Autodesk Inventor part; units mm, degrees
ref_plane "Work Plane2" through (-3.375, 53.625, 0) normal (0, 0, 1) x (1, 0, 0)
ref_plane "YZ Plane" through (0, 0, 0) normal (1, 0, 0) x (0, 1, 0)
ref_plane "XZ Plane" through (0, 0, 0) normal (0, 1, 0) x (-1, 0, 0)
ref_plane "Work Plane1" through (0, 0, 15) normal (0, 0, 1) x (1, 0, 0)
sketch "Sketch1" plane through (0, 0, 15) normal (0, 0, 1) x (1, 0, 0)
  circle A0 centre (0, 64) radius 1.4
  circle A1 centre (0, 0) radius 1.4
  circle A2 centre (38.4621, 0) radius 1.4
  circle A3 centre (76.9242, 0) radius 1.4
  circle A4 centre (76.9242, 64) radius 1.4
  circle A5 centre (38.4621, 64) radius 1.4
  circle A6 centre (-0.5, 56.5) radius 1.375
  circle A7 centre (-0.5, 7.5) radius 1.375
  circle A8 centre (57.5, 7.5) radius 1.375
  circle A9 centre (57.5, 56.5) radius 1.375
  line L0 (0, 68) -> (76.9242, 68)
  arc A10 (80.9242, 64) -> (76.9242, 68) centre (76.9242, 64) ccw
  line L1 (80.9242, 64) -> (80.9242, 0)
  arc A11 (76.9242, -4) -> (80.9242, 0) centre (76.9242, 0) ccw
  line L2 (76.9242, -4) -> (0, -4)
  arc A12 (-4, 0) -> (0, -4) centre (0, 0) ccw
  line L3 (-4, 0) -> (-4, 64)
  arc A13 (0, 68) -> (-4, 64) centre (0, 64) ccw
  line L4 (57.5, 60.619) -> (2.1636, 60.619)
  line L5 (2.1636, 60.619) -> (2.1636, 51.644)
  line L6 (2.1636, 51.644) -> (57.5, 51.644)
  line L7 (57.5, 51.644) -> (57.5, 60.619)
  line L8 (80.9242, 59.8893) -> (61.2665, 59.8893)
  line L9 (61.2665, 59.8893) -> (61.2665, 4.7989)
  line L10 (61.2665, 4.7989) -> (80.9242, 4.7989)
  line L11 (80.9242, 4.7989) -> (80.9242, 59.8893)
  point P0 (0, 0)
extrude "Extrusion1" add sketch "Sketch1" against normal blind 2 contours A6 | A7 | A8 | A9 L7 | L7 A9 | L0 A10 L1 L8 L9 L10 A11 L2 A12 L3 A13
sketch "Sketch2" plane through (0, 0, 13) normal (0, 0, -1) x (-1, 0, 0)
  circle A0 centre (-38.4621, 0) radius 2.9
  circle A1 centre (-38.4621, 64) radius 2.9
  circle A2 centre (0, 0) radius 1.4
  circle A3 centre (-38.4621, 0) radius 1.4
  circle A4 centre (-76.9242, 0) radius 1.4
  circle A5 centre (-76.9242, 64) radius 1.4
  circle A6 centre (-38.4621, 64) radius 1.4
  circle A7 centre (0, 64) radius 1.4
  circle A8 centre (-76.9242, 0) radius 4
  circle A9 centre (-76.9242, 64) radius 4
  circle A10 centre (0, 64) radius 4
  circle A11 centre (0, 0) radius 4
  point P0 (0, 0)
ref_plane "Work Plane2" through (-3.375, 53.625, 0) normal (0, 0, 1) x (1, 0, 0)
extrude "Extrusion2" add sketch "Sketch2" along normal up to surface (13 mm away)
fillet "Fillet1" radius 4 4 edges at (61.2665, 4.7989, 14) (61.2665, 59.8893, 14) (80.9242, 59.8893, 14) (80.9242, 4.7989, 14)
sketch "Sketch3" plane through (0, 0, 15) normal (0, 0, 1) x (1, 0, 0)
  circle A0 centre (46, 6.6021) radius 1.05
  line L0 (48, 30.0021) -> (-9, 30.0021)
  line L1 (-9, 30.0021) -> (-9, 4.6021)
  line L2 (-9, 4.6021) -> (48, 4.6021)
  line L3 (48, 4.6021) -> (48, 30.0021)
  circle A1 centre (-1, 27.9021) radius 1.05
  circle A2 centre (46, 6.6021) radius 1.05
  circle A3 centre (46, 28.0021) radius 1.05
  circle A4 centre (-0.5, 7.5) radius 1.375
  line L4 (43.458, 3.7531) -> (1.4128, 3.7531)
  line L5 (1.4128, 3.7531) -> (1.4128, 8.2423)
  line L6 (1.4128, 8.2423) -> (43.458, 8.2423)
  line L7 (43.458, 8.2423) -> (43.458, 3.7531)
  line L8 (43.458, 31.4547) -> (0.5917, 31.4547)
  line L9 (0.5917, 31.4547) -> (0.5917, 25.5421)
  line L10 (0.5917, 25.5421) -> (43.458, 25.5421)
  line L11 (43.458, 25.5421) -> (43.458, 31.4547)
  point P0 (0, 0)
extrude "Extrusion3" cut sketch "Sketch3" against normal through all contours A0 | L11 L10 L9 L0 | L0 L9 L8 L11 | L7 L4 L5 L2 | L2 L5 L6 L7 | A3
sketch "Sketch4" plane through (0, 0, 15) normal (0, 0, 1) x (1, 0, 0)
  line L0 (76.9242, 68) -> (0, 68)
  line L1 (-4, 64) -> (-4, 0)
  point P0 (0, 0)
  point P1 (28, 63.5)
  point P2 (54, 33.5)
  dimension "d8" = 4.5
  dimension "d9" = 32
  dimension "d10" = 30
  dimension "d11" = 26
hole "Hole1" at (28, 63.5, 15) at (54, 33.5, 15) direction (0, 0, -1) diameter 2.8 depth 20 tip angle 118
properties part number "cellSTORM_v5_Electronicbox_midlayer"
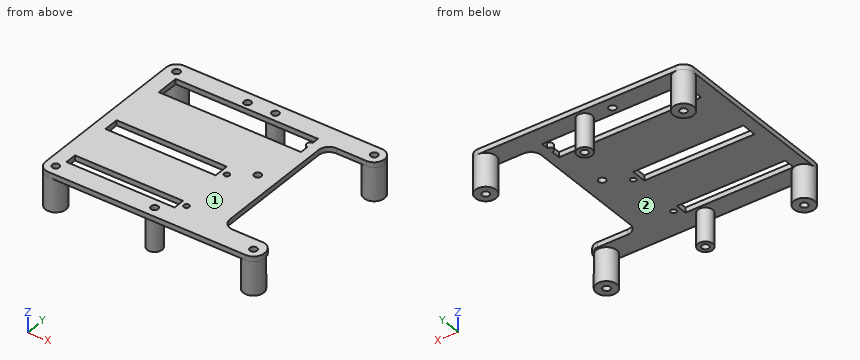
Build history of the part. All positions in model axes, mm. Face numbers are marked on the shaded views. Coordinates: 2 decimals unless noted, no trailing zeros. Write each loop counter-clockwise with the first axis right and the second up, starting at its lowest first coordinate (ties: lowest second). Pieces come first, ordered by that corner, then holes.
(1) Cut at C-C on x = 54. List the corners of the cut face in (y, z), and give its area (3 significant figures).
(2) Pin check, flat tips, straight feed: pin 1 Ø2.5 at (x, y) = (38.46, 64) entering from +Z; pin 2 Ø8 at (x, y) = (52, 20.5) entering from -Z; pin 3 Ø1.6 at (y, z) = (7, 13.5) entering from +X; pin 4 Ø1 at (y, z) = (54, 13.5) entering from +X. Stop position of each tip, or through.
(3) Drill centre lines: line 1 (Y direction, x = 0, z = 13.5); line 2 (X direction, y = 0, z = 13.65); line 3 (Y direction, x = 46, z = 14). Where is each one in solid material? Low to high.
(4) Cut at B-B on z = 7.5. State how many separate pieces and enclosed holes the cut face has, and give its area (3 significant figures).
(5) Cut at D-D on x = 12. List the corners of the cut face in (y, z), and give its area (3 significant figures).
(6) Mould opens along Y. For the marked faces 1 and 2 say: pulls with the +Y half, pulls with the -Y half, needs draft (parallel to the pull), parting line crosses it, or undercut.
(7) Cut at A-A on x = 28. List the corners of the cut face in (y, z), and give its area (3 significant figures).
Working result:
1. outline: (-4, 13) - (32.1, 13) - (32.1, 15) - (-4, 15) - close; (34.9, 13) - (51.64, 13) - (51.64, 15) - (34.9, 15) - close; (60.62, 13) - (68, 13) - (68, 15) - (60.62, 15) - close
1. area: 120 mm2
2. pin 1: passes through
2. pin 2: stops at z = 13
2. pin 3: stops at x = 62.23
2. pin 4: stops at x = 61.27
3. line 1: y = -4 to -1.4, 1.4 to 62.6, 65.4 to 68
3. line 2: x = -4 to -1.4, 1.4 to 37.06, 39.86 to 75.52, 78.32 to 80.92
3. line 3: y = -4 to 5.55, 7.65 to 26.95, 29.05 to 51.64, 60.62 to 68
4. separate pieces: 6
4. enclosed holes: 6
4. area: 217 mm2
5. outline: (-4, 13) - (3.75, 13) - (3.75, 15) - (-4, 15) - close; (8.24, 13) - (25.54, 13) - (25.54, 15) - (8.24, 15) - close; (31.45, 13) - (51.64, 13) - (51.64, 15) - (31.45, 15) - close; (60.62, 13) - (68, 13) - (68, 15) - (60.62, 15) - close
5. area: 105 mm2
6. face 1: needs draft
6. face 2: undercut
7. outline: (-4, 13) - (3.75, 13) - (3.75, 15) - (-4, 15) - close; (8.24, 13) - (25.54, 13) - (25.54, 15) - (8.24, 15) - close; (31.45, 13) - (51.64, 13) - (51.64, 15) - (31.45, 15) - close; (60.62, 13) - (62.1, 13) - (62.1, 15) - (60.62, 15) - close; (64.9, 13) - (68, 13) - (68, 15) - (64.9, 15) - close
7. area: 99.6 mm2
